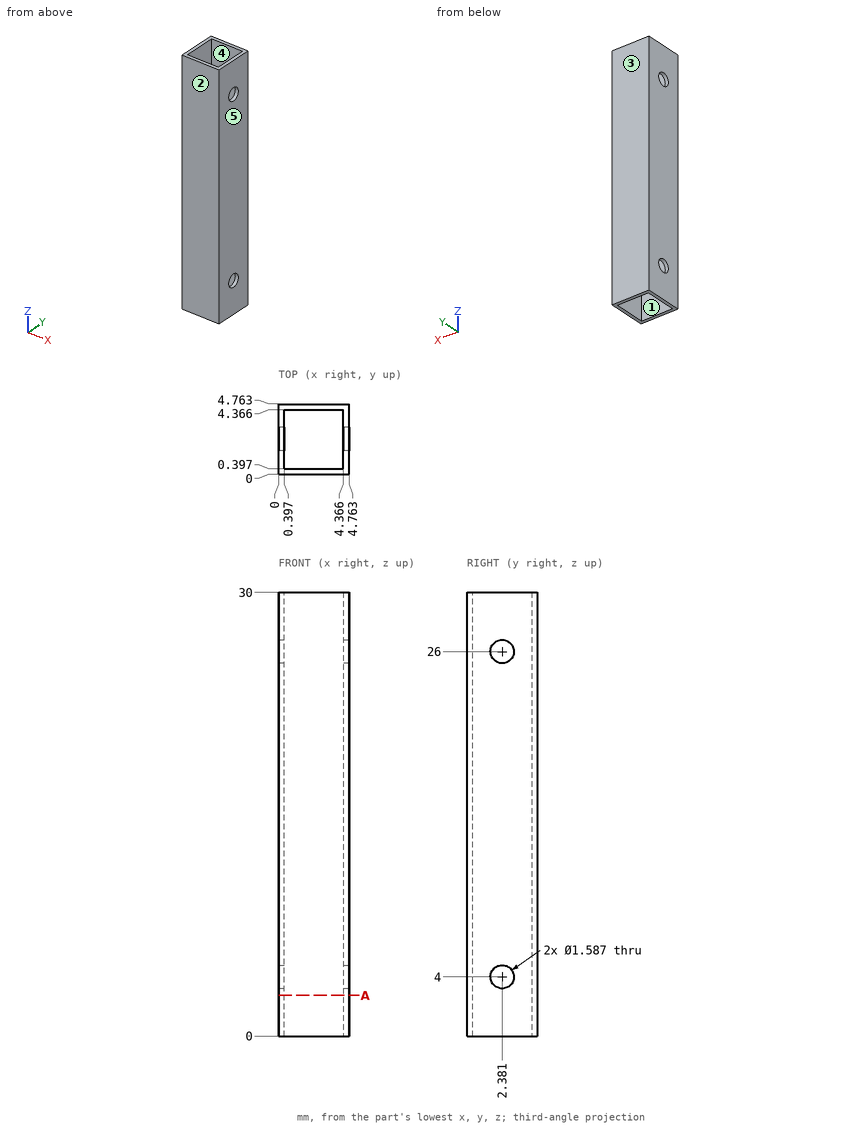
Check sheet for the drawn part. Datum: minimum x, y, z corner. Units: mm. A direction names the side the tool comes from. Coordinates: 2 decimals unless noted, no trailing zeros. Loops run counter-clockwise (first coordinate to the right, second up) from the corner with the lowest first, then second, coordinate; pieces in that order, holes last. Notation, with made-up numbers: (61, -12) - (105, -12) arc R26 cw to (105, 15) - close; hole circle Ø6 at (-18.5, 37.25). An arc over 180 degrees is marked (long way). Put each result on its own line as item: value.
Item 1: Set-up check for the marked faces 1 and 2: record each of +Z, -Z, +X, -X, +Y, -Y from which the full face is reachable in a straight line by a thin tool's end or side.
Conclusion:
face 1: +Z, -Z
face 2: +Z, -Z, +X, -X, -Y
Item 2: Scan lines: line 1 along X through (y, z) = (3.9, 15.75) (1 decimal); line 2 along Y through (x, z) = (4.65, 4) (1 decimal). Record each from-to range of solid material in increasing order.
Conclusion:
line 1: x = 0 to 0.4, 4.4 to 4.8
line 2: y = 0 to 1.6, 3.2 to 4.8
Item 3: Gauge pin test, flat ends, axial feed: pin 1 Ø2 at (y, z) = (2.38, 4) entering from -X; pin 2 Ø1.4 at (y, z) = (2.38, 26) entering from +X. Record the tip position at first contact, or that the pin passes through.
Conclusion:
pin 1: stops at x = 0
pin 2: passes through
Item 4: Section check A-A (z = 2.75). Enter the section's corners in (x, y) (1 decimal).
Conclusion:
outline: (0, 0) - (4.8, 0) - (4.8, 4.8) - (0, 4.8) - close; hole (0.4, 0.4) - (4.4, 0.4) - (4.4, 4.4) - (0.4, 4.4) - close
Item 5: Draft check along X on the marked faces 3, 4 and 5. Enter one of: pulls with the +X half, pulls with the -X half, needs draft (parallel to the pull), parting line crosses it, or undercut.
Conclusion:
face 3: needs draft
face 4: undercut
face 5: pulls with the +X half
